Geometry: see drawing. Coordinates: mm, zero at the bounding-box minimum. A direction names the side the tool comes from. Round coordinates to 2 decimals unless told otherwise and drop trailing zeros. Loops run counter-clockwise (first coordinate to the right, second up) from the corner with the lowest first, then second, coordinate; pieces in that order, holes last. Notation, with made-up numbers: M 13,39.5 L 18,39.5 A18 ccw 18,52.5 Z; hole C -6,21.25 d8. An arc over 180 degrees is marked long. Answer as a JSON object with one key per item and string values.
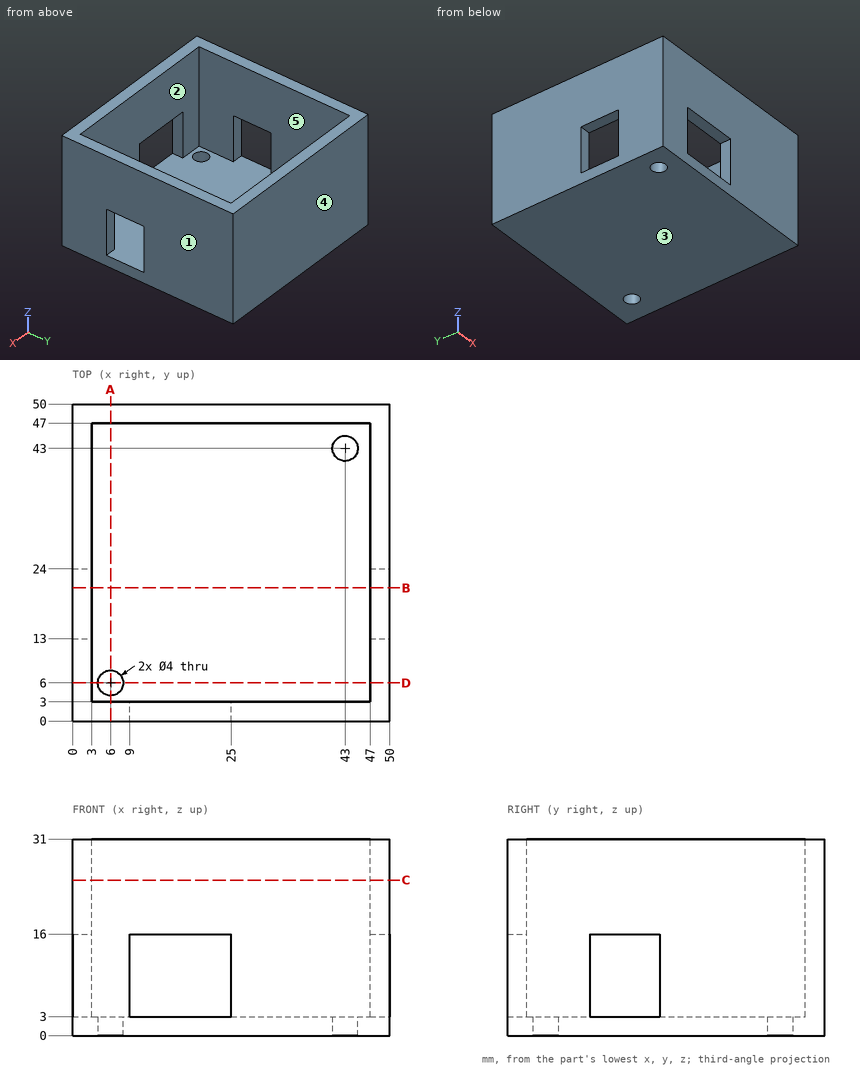
1) Pin query (flat end, axial travel): P1, Ø3.5, axis at y = 2, z = 10.5, coming from the -X side; P2, Ø1.5, axis at x = 14, y = 27.5, coming from the +Z side. Return the tip coordinate at first contact, or that it passes through.
Results:
{"P1": "x = 0", "P2": "z = 3"}
2) Section query C-C (z = 24.5). Return the cut outline in (x, y).
Results:
{"outline": "M 0,0 L 50,0 L 50,50 L 0,50 Z; hole M 3,3 L 47,3 L 47,47 L 3,47 Z"}
3) Pull-direction query (X, two-part tool) for the marked faces 1, 2 and 3; classes: +X half, -X half, draft (parallel to the pull), parting line (faces both ways), or undercut.
Results:
{"face 1": "+X half", "face 2": "undercut", "face 3": "draft"}
4) Section query B-B (y = 21). Return the cut outline in (x, z), and give its area (3 significant figures).
Results:
{"outline": "M 0,0 L 50,0 L 50,3 L 0,3 Z; M 0,16 L 3,16 L 3,31 L 0,31 Z; M 47,16 L 50,16 L 50,31 L 47,31 Z", "area": "240 mm2"}
5) Section query A-A (x = 6). Return the cut outline in (y, z).
Results:
{"outline": "M 0,0 L 4,0 L 4,3 L 3,3 L 3,31 L 0,31 Z; M 8,0 L 50,0 L 50,31 L 47,31 L 47,3 L 8,3 Z"}
6) Reachability of the marked faces 4 and 5 from +Z, -Z, +X, -X, +Y, -Y: full face, straight path, thin tool, end or side. Return the list, or none.
Results:
{"face 4": "+Z, -Z, +X, -X, +Y", "face 5": "+Z"}
7) Ray query, line 1 (X direction, y = 8, z = 13); line 2 (Y direction, x = 43, z = 0.9); line 3 (Y direction, x = 6, z = 2.15). Return the intervals inside material, ascending.
Results:
{"line 1": "0 to 3, 47 to 50", "line 2": "0 to 41, 45 to 50", "line 3": "0 to 4, 8 to 50"}
